Read the model definition and answer for the solid it produces. Units are mm, in the model's axes. Face numbers are marked on the shaded views. A direction names the side the tool comes from. Give positions to 0.01 mm unless a question says otherwise; leave off trailing zeros. Write each loop counter-clockwise with the first axis right and the second up, starting at its lowest first coordinate (ties: lowest second). Pieces come first, ordered by that corner, then holes. Notation, with made-up numbers: (14, 20) - (18, 20) arc R6 cw to (18, 28) - close; hole circle Ø5 at (2.5, -31.75). An arc over 180 degrees is marked (long way). Answer as CSV lines item,"result".
Autodesk Inventor part; units mm, degrees
ref_plane "Work Plane1" through (0, 0, -15) normal (0, 0, 1) x (1, 0, 0)
ref_plane "YZ Plane" through (0, 0, 0) normal (1, 0, 0) x (0, 1, 0)
ref_plane "XZ Plane" through (0, 0, 0) normal (0, 1, 0) x (-1, 0, 0)
sketch "Sketch1" plane through (0, 0, 0) normal (0, 0, 1) x (1, 0, 0)
  line L0 (0, 0) -> (25, 0)
  line L1 (25, 0) -> (25, 40)
  line L2 (25, 40) -> (0, 40)
  line L3 (0, 40) -> (0, 0)
  dimension "d1" = 25
  dimension "d2" = 40
  dimension "d3" = 25
extrude "Extrusion1" add sketch "Sketch1" against normal blind 30
sketch "Sketch2" plane through (25, 0, 0) normal (1, 0, 0) x (0, 0, -1)
  line L0 (0, 0) -> (30, 0)
  circle A0 centre (15, 6.56) radius 2.46
extrude "Extrusion2" cut sketch "Sketch2" against normal blind 30
sketch "Sketch3" plane through (0, 0, 0) normal (-1, 0, 0) x (0, 0, 1)
  line L0 (0, 0) -> (-30, 0)
  line L1 (-25.05, 0) -> (-4.95, 0)
  line L2 (-4.95, 0) -> (-4.95, 33.12)
  line L3 (-4.95, 33.12) -> (-25.05, 33.12)
  line L4 (-25.05, 33.12) -> (-25.05, 0)
  dimension "d11" = 20.1
extrude "Extrusion3" cut sketch "Sketch3" against normal blind 20
sketch "Sketch4" plane through (0, 0, 0) normal (0, -1, 0) x (1, 0, 0)
  line L0 (20, -4.95) -> (20, -25.05)
  line L1 (20, -15) -> (25, -15)
  line L2 (25, 0) -> (25, -30)
  line L3 (20, -8.025) -> (25, -8.025)
  line L4 (25, -8.025) -> (25, -21.975)
  line L5 (25, -21.975) -> (20, -21.975)
  line L6 (20, -21.975) -> (20, -8.025)
  line L7 (20, -8.025) -> (25, -21.975) construction
  line L8 (25, -8.025) -> (20, -21.975) construction
  line L9 (25, -12.54) -> (25, -17.46)
  point P0 (0, 0)
  point P1 (22.5, -15)
  dimension "d14" = 13.95
extrude "Extrusion4" add sketch "Sketch4" along normal blind 15
sketch "Sketch5" plane through (20, 0, 0) normal (-1, 0, 0) x (0, 0, 1)
  circle A0 centre (-15, 6.56) radius 2.46
  circle A1 centre (-15, 6.56) radius 4.7025
  circle A2 centre (-15, 6.56) radius 2.46
  circle A3 centre (-15, 6.56) radius 2.46
  point P0 (0, 0)
  dimension "d17" = 9.405
extrude "Extrusion5" cut sketch "Sketch5" against normal blind 2.1
sketch "Sketch6" plane through (25, 0, 0) normal (1, 0, 0) x (0, 0, -1)
  circle A0 centre (15, 6.56) radius 4.7025
  line L0 (15, 6.56) -> (15, 23.56)
  circle A1 centre (15, 23.56) radius 2.46
  point P0 (0, 0)
  dimension "d20" = 17
  dimension "d21" = 4.92
extrude "Extrusion6" cut sketch "Sketch6" against normal blind 10 contours A1
sketch "Sketch7" plane through (20, 0, 0) normal (-1, 0, 0) x (0, 0, 1)
  circle A0 centre (-15, 23.56) radius 2.46
  circle A1 centre (-15, 23.56) radius 4.7025
  point P0 (0, 0)
  dimension "d24" = 9.405
extrude "Extrusion7" cut sketch "Sketch7" against normal blind 2.1
sketch "Sketch9" plane through (25, 0, 0) normal (1, 0, 0) x (0, 0, -1)
  circle A0 centre (15, 6.56) radius 2.46
  circle A1 centre (15, 6.56) radius 2.46
  circle A2 centre (15, 23.56) radius 2.46
  circle A3 centre (15, 23.56) radius 2.46
  line L0 (30, 40) -> (30, 0)
  line L1 (30, 0) -> (30, 40)
  line L2 (30, 40) -> (0, 40)
  line L3 (0, 40) -> (0, 0)
  line L4 (0, 0) -> (8.025, 0)
  line L5 (21.975, 0) -> (21.975, -15)
  line L6 (21.975, -15) -> (8.025, -15)
  line L7 (8.025, -15) -> (8.025, 0)
  line L8 (0, 0) -> (8.025, 0)
  line L9 (21.975, 0) -> (30, 0)
extrude "Extrusion8" add sketch "Sketch9" along normal blind 5
sketch "Sketch10" plane through (0, 40, 0) normal (0, 1, 0) x (1, 0, 0)
  line L0 (0, 30) -> (30, 30)
  line L1 (30, 0) -> (0, 0)
  line L2 (0, 30) -> (30, 30)
  line L3 (30, 30) -> (30, 0)
  line L4 (30, 0) -> (0, 0)
  line L5 (0, 0) -> (0, 30)
extrude "Extrusion9" add sketch "Sketch10" along normal blind 30
sketch "Sketch12" plane through (30, 0, 0) normal (1, 0, 0) x (0, 0, -1)
  circle A0 centre (15, 6.56) radius 2.46
  line L0 (15, 6.56) -> (15, 15.06)
  circle A1 centre (15, 15.06) radius 2.525
  point P0 (0, 0)
  dimension "d31" = 8.5
  dimension "d33" = 5.05
extrude "Extrusion10" cut sketch "Sketch12" against normal blind 30 contours A1
sketch "Sketch14" plane through (0, 0, 0) normal (0, 0, 1) x (1, 0, 0)
  line L0 (30, 70) -> (0, 70)
  line L1 (0, 100) -> (-8, 100)
  line L2 (30, 0) -> (30, 70)
  line L3 (30, 118) -> (30, 70)
  line L4 (30, 105) -> (30, 100)
  line L5 (0, 70) -> (30, 70)
  line L6 (0, 70) -> (0, 100)
  line L7 (-8, 145) -> (15, 145)
  line L8 (-2, 142.5) -> (-8, 145)
  line L9 (-2, 102.5) -> (-8, 100)
  line L10 (-2, 102.5) -> (4, 122.5)
  line L11 (4, 122.5) -> (-2, 142.5)
  line L12 (15, 145) -> (30, 122.5)
  line L13 (30, 122.5) -> (30, 118)
  point P0 (0, 0)
  dimension "d47" = 30
  dimension "d85" = 45
extrude "Extrusion12" add sketch "Sketch14" against normal blind 30
sketch "Sketch15" plane through (0, 0, -25.05) normal (-1, 0, 0) x (0, 0, 1)
  line L0 (0, 33.12) -> (20.1, 33.12)
  line L1 (20.1, 33.12) -> (20.1, 0)
  line L2 (0, 33.12) -> (20.1, 33.12)
  line L3 (20.1, 33.12) -> (20.1, 31.1)
  line L4 (20.1, 31.1) -> (0, 31.1)
  line L5 (0, 31.1) -> (0, 33.12)
  point P0 (25.05, 0)
  dimension "d57" = 2.02
extrude "Extrusion13" add sketch "Sketch15" against normal blind 20
sketch "Sketch25" plane through (0, 0, 0) normal (0, 0, 1) x (1, 0, 0)
  line L0 (-8, 100) -> (0, 100)
  line L1 (0, 100) -> (-8, 100)
  line L2 (-8, 100) -> (-2, 102.5)
  line L3 (-8, 100) -> (-2, 102.5)
  line L4 (-2, 102.5) -> (4, 122.5)
  line L5 (-8, 145) -> (-2, 142.5)
  line L6 (4, 122.5) -> (-2, 142.5)
  line L7 (-2, 142.5) -> (-8, 145)
  line L8 (15, 145) -> (-8, 145)
  line L9 (-8, 145) -> (15, 145)
  line L10 (15, 145) -> (30, 122.5)
  line L11 (15, 145) -> (30, 122.5)
  line L12 (30, 122.5) -> (30, 92.5)
  line L13 (30, 0) -> (30, 122.5)
  line L14 (30, 92.5) -> (0, 92.5)
  line L15 (0, 0) -> (0, 100)
  line L16 (0, 92.5) -> (0, 100)
  dimension "d88" = 30
extrude "Extrusion14" add sketch "Sketch25" along normal blind 45
ref_plane "Work Plane1" through (0, 0, -15) normal (0, 0, 1) x (1, 0, 0)
mirror "Mirror1" about plane through (0, 0, -15) normal (0, 0, 1) of "Extrusion14"
properties part number "40mm_x_120mm"
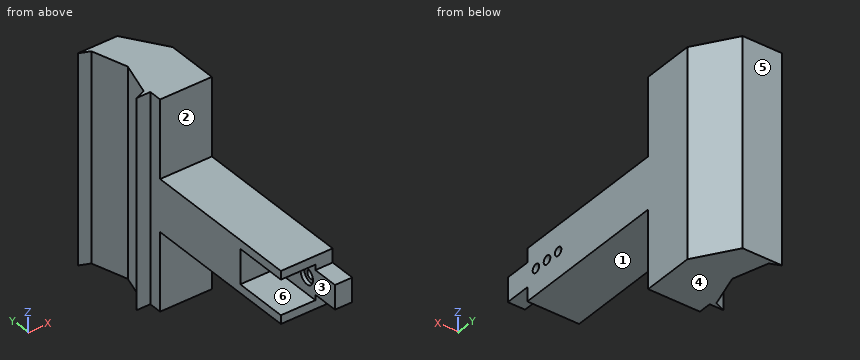
(1) A cutting plane is placed at C-C (x = 13). Write down the section's boundary in (y, z).
Worked out:
outline,"(0, -30) - (92.5, -30) - (92.5, -75) - (145, -75) - (145, 45) - (92.5, 45) - (92.5, 0) - (0, 0) - (0, -4.95) - (31.1, -4.95) - (31.1, -25.05) - (0, -25.05) - close"
(2) Find the intervals of material crossed by L1, parallel to Z at x = 11, y = 7; L2, parallel to Y at x = 21, z = -15 (1 decimal); L3, parallel to Y at x = 21.55, z = -15 (1 decimal), in increasing order.
Worked out:
L1,"z = -30 to -25.05, -4.95 to 0"
L2,"y = -15 to 1.9, 11.3 to 12.5, 17.6 to 18.9, 28.3 to 136"
L3,"y = -15 to 1.9, 11.3 to 12.5, 17.6 to 18.9, 28.3 to 135.2"
(3) Each of these flat-tipped pins is pushed along its axis until it touches: P1, Ø6, axis at y = 15.5, z = -16.5, coming from the -X side; P2, Ø6, axis at x = 12, y = 8, coming from the +Z side; P3, Ø8, axis at y = 16, z = -31.5, coming from the +X side; P4, Ø10, axis at x = 14.5, y = 21.5, coming from the -Z side. Where does it stop, or does it pass through?
Worked out:
P1,"stops at x = 20"
P2,"stops at z = 0"
P3,"stops at x = 30"
P4,"stops at z = -30"
(4) For the marked faces 1, 2 and 3, determine the directions among +Z, -Z, +X, -X, +Y, -Y from which every point of the face is accessible in a straight line to the end or side of a thin tool.
Worked out:
face 1,"-Z, +X, -X, -Y"
face 2,"+Z, +X, -X, -Y"
face 3,"-X, -Y"
(5) A cutting plane is placed at D-D (z = 37.5). Write down the section's boundary in (x, y), and give its area (3 significant figures).
Worked out:
outline,"(-8, 100) - (0, 100) - (0, 92.5) - (30, 92.5) - (30, 122.5) - (15, 145) - (-8, 145) - (-2, 142.5) - (4, 122.5) - (-2, 102.5) - close"
area,"1,390 mm^2"
(6) A cutting plane is placed at B-B (y = 6.56). Write down the section's boundary in (x, z), and give its area (3 significant figures).
Worked out:
outline,"(0, -30) - (30, -30) - (30, -17.46) - (22.1, -17.46) - (22.1, -19.7) - (20, -19.7) - (20, -25.05) - (0, -25.05) - close; (0, -4.95) - (20, -4.95) - (20, -10.3) - (22.1, -10.3) - (22.1, -12.54) - (30, -12.54) - (30, 0) - (0, 0) - close"
area,"439 mm^2"
(7) A cutting plane is placed at A-A (z = -15). Count the separate pieces of the cut face and the enclosed holes in it, and give its area (3 significant figures).
Worked out:
separate pieces,"4"
enclosed holes,"0"
area,"3,530 mm^2"
(8) The mould has two halves that part along Z. Classify the marked faces 4, 5 and 6: +Z half, -Z half, draft (parallel to the pull), parting line (faces both ways), or undercut.
Worked out:
face 4,"-Z half"
face 5,"draft"
face 6,"undercut"
